Can you work these out from the model? Positions are in its coordinate system, mm. Coordinates: 2 decimals unless noted, no trailing zeros. Order: outer loops, then holes, each group sorted by start corner. A loop starts at its lowest first (then second) coordinate and runs counter-clockwise, first axis right, second up. Notation, with made-up numbers: (-23, -39) - (18, -39) arc R16 ccw to (18, -25) - close; hole circle Ø2 at (84, -15.5). An arc over 180 degrees is marked (long way). Use a Markdown table: item, result. Add a question column.
(1) For pin 1 Ø0.8 at (y, z) = (-87, 0.5) entering from +X; pin 2 Ø3 at (x, y) = (-7.3, -80) entering from -Z; pin 3 Ø0.5 at (x, z) = (-2, 0.5) entering from +Y, each with a flat end and sliding along its axis, tell me the tip position at first contact or that it passes through.
(2) I want a section at A-A (x = -77). List the corners of the cut face in (y, z) for me, and give its area (3 significant figures).
(3) If I drill on L1, parallel to X at y = -33, z = 1.25 (3 decimals), over which ranges is the centre line in solid material (lowest first)? Write a range as [from, to].
```python
from build123d import *

# Parameters (mm, degrees)
SKETCH1_R           = 1.9
SKETCH1_R_2         = 0.375
SKETCH1_R_3         = 0.383755901
SKETCH1_R_4         = 0.384163196
SKETCH1_R_5         = 0.380771211
SKETCH1_R_6         = 0.377379225
SKETCH1_R_7         = 0.380832793
BOSS_EXTRUDE1_DEPTH = 1.6


with BuildPart() as part:
    # Sketch1 → Boss-Extrude1 (new body)
    with BuildSketch(Plane.XY):
        Polygon((-3, 0), (-86, 0), (-86, -90), (-3, -90), (-3, -85), (0, -85), (0, -5), (-3, -5), align=None)
        with Locations((-7.3, -10)):
            Circle(SKETCH1_R, mode=Mode.SUBTRACT)
        with Locations((-77.3, -10)):
            Circle(SKETCH1_R, mode=Mode.SUBTRACT)
        with Locations((-77.3, -80)):
            Circle(SKETCH1_R, mode=Mode.SUBTRACT)
        with Locations((-7.3, -80)):
            Circle(SKETCH1_R, mode=Mode.SUBTRACT)
        with Locations((-9.3, -69)):
            Circle(SKETCH1_R_2, mode=Mode.SUBTRACT)
        with Locations((-7.3, -69)):
            Circle(SKETCH1_R_2, mode=Mode.SUBTRACT)
        with Locations((-7.3, -67)):
            Circle(SKETCH1_R_2, mode=Mode.SUBTRACT)
        with Locations((-9.3, -67)):
            Circle(SKETCH1_R_2, mode=Mode.SUBTRACT)
        with Locations((-9.3, -65)):
            Circle(SKETCH1_R_2, mode=Mode.SUBTRACT)
        with Locations((-7.3, -65)):
            Circle(SKETCH1_R_2, mode=Mode.SUBTRACT)
        with Locations((-7.3, -63)):
            Circle(SKETCH1_R_2, mode=Mode.SUBTRACT)
        with Locations((-9.3, -63)):
            Circle(SKETCH1_R_3, mode=Mode.SUBTRACT)
        with Locations((-9.3, -61)):
            Circle(SKETCH1_R_2, mode=Mode.SUBTRACT)
        with Locations((-7.3, -61)):
            Circle(SKETCH1_R_2, mode=Mode.SUBTRACT)
        with Locations((-7.3, -59)):
            Circle(SKETCH1_R_2, mode=Mode.SUBTRACT)
        with Locations((-9.3, -59)):
            Circle(SKETCH1_R_2, mode=Mode.SUBTRACT)
        with Locations((-7.3, -57)):
            Circle(SKETCH1_R_2, mode=Mode.SUBTRACT)
        with Locations((-9.3, -57)):
            Circle(SKETCH1_R_2, mode=Mode.SUBTRACT)
        with Locations((-9.3, -55)):
            Circle(SKETCH1_R_2, mode=Mode.SUBTRACT)
        with Locations((-7.3, -55)):
            Circle(SKETCH1_R_2, mode=Mode.SUBTRACT)
        with Locations((-7.3, -53)):
            Circle(SKETCH1_R_2, mode=Mode.SUBTRACT)
        with Locations((-9.3, -53)):
            Circle(SKETCH1_R_2, mode=Mode.SUBTRACT)
        with Locations((-9.3, -51)):
            Circle(SKETCH1_R_2, mode=Mode.SUBTRACT)
        with Locations((-7.3, -51)):
            Circle(SKETCH1_R_2, mode=Mode.SUBTRACT)
        with Locations((-7.3, -49)):
            Circle(SKETCH1_R_2, mode=Mode.SUBTRACT)
        with Locations((-9.3, -49)):
            Circle(SKETCH1_R_2, mode=Mode.SUBTRACT)
        with Locations((-9.3, -47)):
            Circle(SKETCH1_R_2, mode=Mode.SUBTRACT)
        with Locations((-7.3, -47)):
            Circle(SKETCH1_R_2, mode=Mode.SUBTRACT)
        with Locations((-7.3, -45)):
            Circle(SKETCH1_R_2, mode=Mode.SUBTRACT)
        with Locations((-9.3, -45)):
            Circle(SKETCH1_R_4, mode=Mode.SUBTRACT)
        with Locations((-9.3, -43)):
            Circle(SKETCH1_R_2, mode=Mode.SUBTRACT)
        with Locations((-7.3, -43)):
            Circle(SKETCH1_R_5, mode=Mode.SUBTRACT)
        with Locations((-7.3, -41)):
            Circle(SKETCH1_R_6, mode=Mode.SUBTRACT)
        with Locations((-9.3, -41)):
            Circle(SKETCH1_R_6, mode=Mode.SUBTRACT)
        with Locations((-9.3, -39)):
            Circle(SKETCH1_R_2, mode=Mode.SUBTRACT)
        with Locations((-7.3, -39)):
            Circle(SKETCH1_R_2, mode=Mode.SUBTRACT)
        with Locations((-7.3, -37)):
            Circle(SKETCH1_R_2, mode=Mode.SUBTRACT)
        with Locations((-9.3, -37)):
            Circle(SKETCH1_R_7, mode=Mode.SUBTRACT)
        with Locations((-7.3, -35)):
            Circle(SKETCH1_R_2, mode=Mode.SUBTRACT)
        with Locations((-9.3, -35)):
            Circle(SKETCH1_R_2, mode=Mode.SUBTRACT)
        with Locations((-9.3, -33)):
            Circle(SKETCH1_R_2, mode=Mode.SUBTRACT)
        with Locations((-7.3, -33)):
            Circle(SKETCH1_R_2, mode=Mode.SUBTRACT)
        with Locations((-7.3, -31)):
            Circle(SKETCH1_R_2, mode=Mode.SUBTRACT)
        with Locations((-9.3, -31)):
            Circle(SKETCH1_R_2, mode=Mode.SUBTRACT)
        with Locations((-7.3, -29)):
            Circle(SKETCH1_R_2, mode=Mode.SUBTRACT)
        with Locations((-9.3, -29)):
            Circle(SKETCH1_R_2, mode=Mode.SUBTRACT)
        with Locations((-9.3, -27)):
            Circle(SKETCH1_R_2, mode=Mode.SUBTRACT)
        with Locations((-7.3, -27)):
            Circle(SKETCH1_R_2, mode=Mode.SUBTRACT)
        with Locations((-7.3, -25)):
            Circle(SKETCH1_R_2, mode=Mode.SUBTRACT)
        with Locations((-9.3, -25)):
            Circle(SKETCH1_R_2, mode=Mode.SUBTRACT)
        with Locations((-7.3, -23)):
            Circle(SKETCH1_R_2, mode=Mode.SUBTRACT)
        with Locations((-9.3, -23)):
            Circle(SKETCH1_R_2, mode=Mode.SUBTRACT)
        with Locations((-9.3, -21)):
            Circle(SKETCH1_R_2, mode=Mode.SUBTRACT)
        with Locations((-7.3, -21)):
            Circle(SKETCH1_R_2, mode=Mode.SUBTRACT)
    extrude(amount=BOSS_EXTRUDE1_DEPTH)


solid = part.part
```
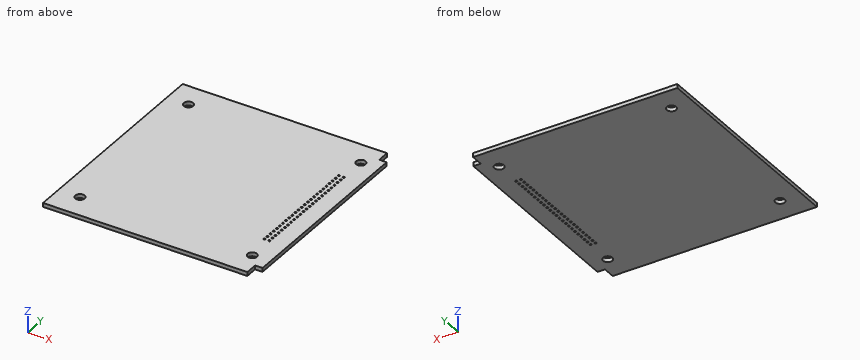
Answers follow:
| question | item | result |
|---|---|---|
| 1 | pin 1 | stops at x = -3 |
| 1 | pin 2 | passes through |
| 1 | pin 3 | stops at y = -5 |
| 2 | outline | (-90, 0) - (-81.88, 0) - (-81.88, 1.6) - (-90, 1.6) - close; (-78.12, 0) - (-11.88, 0) - (-11.88, 1.6) - (-78.12, 1.6) - close; (-8.12, 0) - (0, 0) - (0, 1.6) - (-8.12, 1.6) - close |
| 2 | area | 132 mm² |
| 3 | L1 | x = [-86, -9.675], [-8.925, -7.675], [-6.925, 0] |
